Geometry check sheet. Reference: the model listing, model coordinates, mm. A direction names the side the tool comes from. Coordinates: 2 decimals unless noted, no trailing zeros. Write each loop counter-clockwise with the first axis right and the second up, starting at its lowest first coordinate (ties: lowest second). Pieces come first, ordered by that corner, then holes. Notation, with made-up numbers: M -29.75,74 L -3.75,74 A18 cw -3.75,109 Z; hole C 47.25,74 d11. An arc over 180 degrees is marked long. Answer as a JSON object with one key per item and string values. Group by question number.
```python
from build123d import *

# Parameters (mm, degrees)
BOSS_EXTRUDE1_DEPTH = 25
CHAMFER1_SIZE       = 1
FILLET1_R           = 2


with BuildPart() as part:
    # Sketch1 → Boss-Extrude1 (new body)
    with BuildSketch(Plane(origin=(0, 0, 0), x_dir=(1, 0, 0), z_dir=(0, 1, 0))):
        Polygon((0, 0), (0, -56), (-4, -56), (-4, 0), (-4, 4), (56, 4), (56, 0), align=None)
    extrude(amount=BOSS_EXTRUDE1_DEPTH)

    # Chamfer1
    chamfer1_edges = [part.edges().sort_by_distance(p)[0] for p in [
        (28, 0, 0),
        (26, 25, -4),
        (-4, 25, 26),
        (-2, 25, 56),
        (0, 25, 28),
        (28, 25, 0),
        (0, 0, 28),
        (-2, 0, 56),
        (-4, 0, 26),
        (56, 25, -2),
        (26, 0, -4),
        (56, 0, -2),
    ]]
    chamfer(chamfer1_edges, length=CHAMFER1_SIZE)

    # Fillet1
    fillet1_edges = [part.edges().sort_by_distance(p)[0] for p in [
        (-4, 12.5, -4),
    ]]
    fillet(fillet1_edges, radius=FILLET1_R)


solid = part.part
```
1) Material ranges on probe 1 along X at (y, z) = (19, 4); probe 2 along Y at (x, z) = (44, -0.5), recorded low to high. Write a range as [from, to].
2) Set-up check for faces 1 (the flat face through (-4, 12, 27)), 2 (the flat face through (28, 12, 0)): record each of +Z, -Z, +X, -X, +Y, -Y from which the full face is reachable in a straight line by a thin tool's end or side.
3) Go/stop test with flat-tipped pins: pin 1 Ø5 at (y, z) = (10.5, 11.5) entering from +X; pin 2 Ø8 at (x, y) = (36, 11) entering from +Z. Record where each tip stops, or that it passes through.
4) Section check B-B (z = 14.5). Record the cut outline in (x, y), then the cut area to 3 significant figures.
5) Section check C-C (x = 38). Record the cut outline in (y, z).
6) Section check A-A (y = 11.75). Record the cut outline in (x, z), then the cut area to 3 significant figures.
Entries:
{
 "1": {"probe 1": "[-4, 0]", "probe 2": "[0.5, 24.5]"},
 "2": {"face 1": "+Z, -Z, -X, +Y, -Y", "face 2": "+Z, +X, +Y, -Y"},
 "3": {"pin 1": "x = 0", "pin 2": "z = 0"},
 "4": {"outline": "M -4,1 L -3,0 L -1,0 L 0,1 L 0,24 L -1,25 L -3,25 L -4,24 Z", "area": "98.0 mm^2"},
 "5": {"outline": "M 0,-3 L 1,-4 L 24,-4 L 25,-3 L 25,-1 L 24,0 L 1,0 L 0,-1 Z"},
 "6": {"outline": "M -4,-2 A2 ccw -2,-4 L 56,-4 L 56,0 L 0,0 L 0,56 L -4,56 Z", "area": "463 mm^2"}
}
